```python
from build123d import *

# Parameters (mm, degrees)
SKETCH_1_R               = 22.5
EXTRUDE_1_DEPTH          = 12
CUT_EXTRUDE_1_DEPTH      = 10
HOLE_WIZARD_M10_1_D      = 8.5
HOLE_WIZARD_M10_1_DEPTH  = 24.5
HOLE_WIZARD_M10_1_TIP    = 2.553657631
PATTERN_CIRCULAR_1_COUNT = 4


with BuildPart() as part:
    # 草图1 → 凸台-拉伸1 (new body)
    with BuildSketch(Plane.XY):
        Circle(SKETCH_1_R)
    extrude(amount=EXTRUDE_1_DEPTH)

    # 草图2 → 切除-拉伸1 (cut)
    with BuildSketch(Plane.XY.offset(12)):
        with BuildLine():
            Line((-18.5, 12.806248475), (-18.5, -12.806248475))
            ThreePointArc((-18.5, -12.806248475), (-22.5, 0), (-18.5, 12.806248475))
        make_face()
        with BuildLine():
            Line((18.5, 12.806248475), (18.5, -12.806248475))
            ThreePointArc((18.5, -12.806248475), (22.5, 0), (18.5, 12.806248475))
        make_face()
    extrude(amount=-CUT_EXTRUDE_1_DEPTH, mode=Mode.SUBTRACT)

    # M10 螺纹孔1
    with Locations(Plane.XY.offset(12)):
        with Locations((0, 0)):
            Hole(HOLE_WIZARD_M10_1_D / 2, depth=HOLE_WIZARD_M10_1_DEPTH)
            with Locations((0, 0, -(HOLE_WIZARD_M10_1_DEPTH + HOLE_WIZARD_M10_1_TIP / 2))):  # 118° drill point
                Cone(0, HOLE_WIZARD_M10_1_D / 2, HOLE_WIZARD_M10_1_TIP, mode=Mode.SUBTRACT)

    # 草图7 → M4 螺纹孔2 (revolve, cut)
    with BuildSketch(Plane(origin=(-12.02081528, 12.02081528, 0), x_dir=(0, 1, 0), z_dir=(1, 0, 0))):
        Polygon((0, 0), (0, 11.091420021), (1.65, 10.1), (1.65, 0), align=None)
    hole_wizard_m4_2 = revolve(axis=Axis((-12.02081528, 12.02081528, -6.35), (0, 0, 1)), mode=Mode.SUBTRACT)

    # 阵列(圆周)1: M4 螺纹孔2 ×4 about axis
    pattern_circular_1_axis = Axis((0, 0, 0), (0, 0, 1))
    for i in range(1, PATTERN_CIRCULAR_1_COUNT):
        add(hole_wizard_m4_2.rotate(pattern_circular_1_axis, i * 360 / PATTERN_CIRCULAR_1_COUNT), mode=Mode.SUBTRACT)


solid = part.part
```
Part model, mm, in its own coordinate system. A direction names the side the tool comes from. Give positions to 0.01 mm unless a question says otherwise; leave off trailing zeros. Order: outer loops, then holes, each group sorted by start corner. A loop starts at its lowest first (then second) coordinate and runs counter-clockwise, first axis right, second up. Notation, with made-up numbers: (24, 28.25) - (33, 28.25) arc R19 cw to (33, 59.25) - close; hole circle Ø11 at (82.5, 24.25). An arc over 180 degrees is marked (long way). Use one line per item in the form item = value.
Item 1: Slice it at A-A on y = 0. Give the cut face in (x, z), and give its area (3 significant figures).
Solution:
outline = (-22.5, 0) - (-4.25, 0) - (-4.25, 12) - (-18.5, 12) - (-18.5, 2) - (-22.5, 2) - close; (4.25, 0) - (22.5, 0) - (22.5, 2) - (18.5, 2) - (18.5, 12) - (4.25, 12) - close
area = 358 mm2
Item 2: Slice it at D-D on y = -5. Give the cut face in (x, z).
Solution:
outline = (-21.94, 0) - (21.94, 0) - (21.94, 2) - (18.5, 2) - (18.5, 12) - (-18.5, 12) - (-18.5, 2) - (-21.94, 2) - close
Item 3: Pin check, flat tips, straight feed: pin 1 Ø4.5 at (x, y) = (20.5, 1) entering from +Z; pin 2 Ø1 at (y, z) = (-2, 1.5) entering from +X; pin 3 Ø5 at (x, z) = (-4, 4.5) entering from +Y; pin 4 Ø1 at (y, z) = (-14, 1.5) entering from +X. Stop position of each tip, or through.
Solution:
pin_1 = 12
pin_2 = 22.45
pin_3 = 22.45
pin_4 = 18
Item 4: Two-plate mould, pull along X, no slides. Class faces 1 (the face through (12, -11.7, 10.9)), 2 (the face through (-4.4, 0.3, 12)), 3 (the face through (-22.48, 0.99, 0.58)): released by +X, released by -X, zero draft, split by the parting line, or undercut.
Solution:
face_1 = undercut
face_2 = zero draft
face_3 = split by the parting line
Item 5: Slice it at B-B on x = 0. Give the cut face in (y, z), and give its area (3 significant figures).
Solution:
outline = (-22.5, 0) - (-4.25, 0) - (-4.25, 12) - (-22.5, 12) - close; (4.25, 0) - (22.5, 0) - (22.5, 12) - (4.25, 12) - close
area = 438 mm2
Item 6: Probe probe 1 along Y at (x, z) = (0, 8.25); probe 2 along Y at (x, z) = (12, 1.5); probe 3 along Y at (x, z) = (11, 9). List the from-to ranges inside material, lowest first. Write a range as from..to.
Solution:
probe_1 = -22.5..-4.25, 4.25..22.5
probe_2 = -19.03..-13.67, -10.37..10.37, 13.67..19.03
probe_3 = -19.63..-13.32, -10.72..10.72, 13.32..19.63
Item 7: Which spindle directions (+Z, -Z, +X, -X, +Y, -Y) get a long thin tool onto all of the face, cutting with end or side? Do faces 4 (the face through (-20, 0, 2)), 5 (the face through (-2.285, 3.584, 5.916)), 6 (the face through (10.71, 11.02, 4.98)), 7 (the face through (20, 0, 2)), 8 (the face through (0, -5, 0)). Say none if no direction does.
Solution:
face_4 = +Z, -X, +Y, -Y
face_5 = +Z, -Z
face_6 = -Z
face_7 = +Z, +X, +Y, -Y
face_8 = -Z, +X, -X, +Y, -Y
Item 8: Slice it at C-C on z = 3.25. Give the cut face in (x, y).
Solution:
outline = (-18.5, -12.81) arc R22.5 ccw to (18.5, -12.81) - (18.5, 12.81) arc R22.5 ccw to (-18.5, 12.81) - close; hole circle Ø3.3 at (-12.02, -12.02); hole circle Ø3.3 at (-12.02, 12.02); hole circle Ø8.5 at (0, 0); hole circle Ø3.3 at (12.02, -12.02); hole circle Ø3.3 at (12.02, 12.02)
